from build123d import *

# Parameters (mm, degrees)
SKETCH2_W                          = 36
SKETCH2_H                          = 25
BOSS_EXTRUDE1_DEPTH                = 24
CUT_EXTRUDE1_DEPTH                 = 12.6
TAP_DRILL_FOR_M2_5X0_45_TAP1_D     = 2.05
TAP_DRILL_FOR_M2_5X0_45_TAP1_DEPTH = 6
FILLET2_R                          = 5
CBORE_FOR_M2_5_SHCS1_D             = 3
CBORE_FOR_M2_5_SHCS1_CBORE_D       = 5.5
CBORE_FOR_M2_5_SHCS1_CBORE_DEPTH   = 4
SKETCH8_W                          = 8
SKETCH8_H                          = 10
CUT_EXTRUDE2_DEPTH                 = 10
FILLET3_R                          = 5


with BuildPart() as part:
    # Sketch2 → Boss-Extrude1 (new body)
    with BuildSketch(Plane(origin=(0, 0, 0), x_dir=(1, 0, 0), z_dir=(0, 1, 0))):
        with Locations((18, 12.5)):
            Rectangle(SKETCH2_W, SKETCH2_H)
    extrude(amount=BOSS_EXTRUDE1_DEPTH)

    # Sketch3 → Cut-Extrude1 (cut)
    with BuildSketch(Plane(origin=(0, 24, 0), x_dir=(1, 0, 0), z_dir=(0, 1, 0))):
        Polygon((6.5, 25), (29.5, 25), (29.5, 9.1), (6.5, 9.1), (5.5, 9.1), (5.5, 14.1), (6.5, 14.1), align=None)
    extrude(amount=-CUT_EXTRUDE1_DEPTH, mode=Mode.SUBTRACT)

    # Tap Drill for M2.5x0.45 Tap1
    with Locations(Plane(origin=(0, 0, -25), x_dir=(-1, 0, 0), z_dir=(0, 0, -1))):
        with Locations((-32.5, 17.7), (-3.5, 17.7)):
            Hole(TAP_DRILL_FOR_M2_5X0_45_TAP1_D / 2, depth=TAP_DRILL_FOR_M2_5X0_45_TAP1_DEPTH)

    # Fillet2
    fillet2_edges = [part.edges().sort_by_distance(p)[0] for p in [
        (36, 12, 0),
    ]]
    fillet(fillet2_edges, radius=FILLET2_R)

    # CBORE for M2.5 SHCS1 (through all)
    with Locations(Plane(origin=(0, 24, 0), x_dir=(1, 0, 0), z_dir=(0, 1, 0))):
        with Locations((30.5, 5), (5.5, 5)):
            CounterBoreHole(CBORE_FOR_M2_5_SHCS1_D / 2, CBORE_FOR_M2_5_SHCS1_CBORE_D / 2, CBORE_FOR_M2_5_SHCS1_CBORE_DEPTH)

    # Sketch8 → Cut-Extrude2 (cut)
    with BuildSketch(Plane.ZY):
        with Locations((-13.1, 19)):
            Rectangle(SKETCH8_W, SKETCH8_H)
    extrude(amount=-CUT_EXTRUDE2_DEPTH, mode=Mode.SUBTRACT)

    # Fillet3
    fillet3_edges = [part.edges().sort_by_distance(p)[0] for p in [
        (0, 12, 0),
    ]]
    fillet(fillet3_edges, radius=FILLET3_R)


solid = part.part
For this review, take the finished solid that the model builds, in its own axes (mm). A direction names the side the tool comes from. Give positions to 0.01 mm unless a question says otherwise; leave off trailing zeros. Loops run counter-clockwise (first coordinate to the right, second up) from the corner with the lowest first, then second, coordinate; pieces in that order, holes last. Notation, with made-up numbers: M 13.25,67.25 L 59.25,67.25 A22 ccw 59.25,77.25 Z; hole C 63.5,39.25 d5. An arc over 180 degrees is marked long. Answer as a JSON object with one key per item and string values. Group by question number.
Q1. Add section A-A on y = 17.7. Give the boundary of the cut face in (x, z) (3 decimals), and give its area (3 significant figures).
Q2. Add section D-D on x = 14.5. Give the boundary of the cut face in (y, z).
Q3. Add section B-B on z = -19.75. Give the boundary of the cut face in (x, y) (3 decimals).
Q4. Insertion check: P1, Ø3.5, axis at x = 30.5, z = -5, coming from the +Y side; P2, Ø8, axis at x = 13, z = -17, coming from the +Y side; P3, Ø1.8, axis at x = 3.5, y = 17.7, coming from the +Z side; P4, Ø1.8, axis at x = 5.5, z = -5, coming from the -Y side. Each pin has a flat end and moves straight along its axis. Give the tip position at first contact, or say it passes through.
Q5. Tool access review of faces 1 (the flat face through (18, 9, -25)), 2 (the flat face through (32, 18, -19)), 3 (the flat face through (3, 14, -13)), 4 (the cylindrical face through (8.04, 22.03, -3.95)), 5 (the cylindrical face through (32, 10, -5)): name each direction out of +Z, -Z, +X, -X, +Y, -Y from which nothing blocks a thin tool from reaching the whole face with its end or side.
Q6. Mouldability with a two-part tool opening along Z and no side actions: class faces 6 (the cylindrical face through (2, 12, -1)), 7 (the flat face through (7, 20, -4)), 8 (the flat face through (29.5, 18, -17)) as +Z half, -Z half, draft (parallel to the pull), parting line (faces both ways), or undercut.
Q7. For probe 1 along Z at (x, y) = (30.5, 13.75); probe 2 along X at (y, z) = (11.75, -15); probe 3 along Z at (x, y) = (30.5, 22), list the stretches that pass through material, from the lowest coordinate up. Write a range as [from, to].
Q8. Add section C-C on y = 12.5. Give the boundary of the cut face in (x, z).
Checked values:
{
 "1": {"outline": "M 0,-25 L 2.475,-25 L 2.475,-19 L 4.525,-19 L 4.525,-25 L 6.5,-25 L 6.5,-17.1 L 0,-17.1 Z; M 0,-9.1 L 29.5,-9.1 L 29.5,-25 L 31.475,-25 L 31.475,-19 L 33.525,-19 L 33.525,-25 L 36,-25 L 36,-5 A5 ccw 31,0 L 5,0 A5 ccw 0,-5 Z; hole C 5.5,-5 d3; hole C 30.5,-5 d3", "area": "433 mm²"},
 "2": {"outline": "M 0,-25 L 11.4,-25 L 11.4,-9.1 L 24,-9.1 L 24,0 L 0,0 Z"},
 "3": {"outline": "M 0,0 L 36,0 L 36,24 L 29.5,24 L 29.5,11.4 L 6.5,11.4 L 6.5,24 L 0,24 Z; hole C 3.5,17.7 d2.05; hole C 32.5,17.7 d2.05"},
 "4": {"P1": "y = 20", "P2": "y = 11.4", "P3": "z = -0.04", "P4": "through"},
 "5": {"face 1": "-Z, +X, -X, +Y, -Y", "face 2": "-Z", "face 3": "-X, +Y", "face 4": "+Y", "face 5": "+Y, -Y"},
 "6": {"face 6": "+Z half", "face 7": "undercut", "face 8": "draft"},
 "7": {"probe 1": "[-25, -6.5], [-3.5, 0]", "probe 2": "[0, 6.5], [29.5, 36]", "probe 3": "[-25, -7.75], [-2.25, 0]"},
 "8": {"outline": "M 0,-25 L 6.5,-25 L 6.5,-14.1 L 5.5,-14.1 L 5.5,-9.1 L 29.5,-9.1 L 29.5,-25 L 36,-25 L 36,-5 A5 ccw 31,0 L 5,0 A5 ccw 0,-5 Z; hole C 5.5,-5 d3; hole C 30.5,-5 d3"}
}
